Build history of the part. All positions in model axes, mm. Face numbers are marked on the shaded views. A direction names the side the tool comes from. Coordinates: 2 decimals unless noted, no trailing zeros. Order: outer loops, then holes, each group sorted by start corner. A loop starts at its lowest first (then second) coordinate and runs counter-clockwise, first axis right, second up. Notation, with made-up numbers: M 33.5,56 L 92.5,56 A20 cw 92.5,82 Z; hole C -32.5,73.5 d10. An arc over 180 degrees is marked long. Write item = value, one per line. Start each with the question number.
Q1. Pin check, flat tip, straight feed: P1, Ø5, axis at x = 4, z = 4, coming from the +Y side. Stop position of the tip, or through.
Q2. 3-axis set-ups, long thin cutter, end or side, ignore diameter. For the marked faces 1 and 2: which of +Z, -Z, +X, -X, +Y, -Y reach the whole face in a straight line?
Q3. Band-saw the part on D-D on x = 12.25. Write the cut outline in (y, z), plus the area to 3 significant figures.
Q4. Pull direction Z, two halves, no side cores. Call the marked faces 3, 4, 5 and 6: released by +Z, released by -Z, zero draft, split by the parting line, or undercut.
Q5. Band-saw the part on A-A on y = 9.25. Write the cut outline in (x, z), plus the area to 3 significant figures.
Q6. Band-saw the part on C-C on z = 4.25. Write the cut outline in (x, y), plus the area to 3 significant figures.
Q7. Drill centre lines: probe 1 along Z at (x, y) = (6.25, 6); probe 2 along Y at (x, z) = (6.35, 8); probe 3 along Y at (x, z) = (3, 1.25). Where is each one in solid material? Low to high.
Q8. Band-saw the part on B-B on x = 6.35. Write the cut outline in (y, z).
```python
from build123d import *

# Parameters (mm, degrees)
SKETCH1_R           = 0.5
BOSS_EXTRUDE1_DEPTH = 1
SKETCH2_W           = 12.7
SKETCH2_H           = 1
BOSS_EXTRUDE2_DEPTH = 6.35
SKETCH3_R           = 0.5
BOSS_EXTRUDE3_DEPTH = 1


with BuildPart() as part:
    # Sketch1 → Boss-Extrude1 (new body)
    with BuildSketch(Plane.XY):
        with BuildLine():
            Line((0, 0), (0, 19.05))
            ThreePointArc((0, 19.05), (6.35, 25.4), (12.7, 19.05))
            Line((12.7, 19.05), (12.7, 0))
            Line((12.7, 0), (0, 0))
        make_face()
        with Locations((6.35, 19.05)):
            Circle(SKETCH1_R, mode=Mode.SUBTRACT)
    extrude(amount=BOSS_EXTRUDE1_DEPTH)

    # Sketch2 → Boss-Extrude2 (add)
    with BuildSketch(Plane.XY.offset(1)):
        with Locations((6.35, 0.5)):
            Rectangle(SKETCH2_W, SKETCH2_H)
    extrude(amount=BOSS_EXTRUDE2_DEPTH)

    # Sketch3 → Boss-Extrude3 (add)
    with BuildSketch(Plane.XY.offset(7.35)):
        with BuildLine():
            Line((0, 0), (12.7, 0))
            Line((12.7, 0), (12.7, 19.05))
            ThreePointArc((12.7, 19.05), (6.35, 25.4), (0, 19.05))
            Line((0, 19.05), (0, 0))
        make_face()
        with Locations((6.35, 19.05)):
            Circle(SKETCH3_R, mode=Mode.SUBTRACT)
    extrude(amount=BOSS_EXTRUDE3_DEPTH)


solid = part.part
```
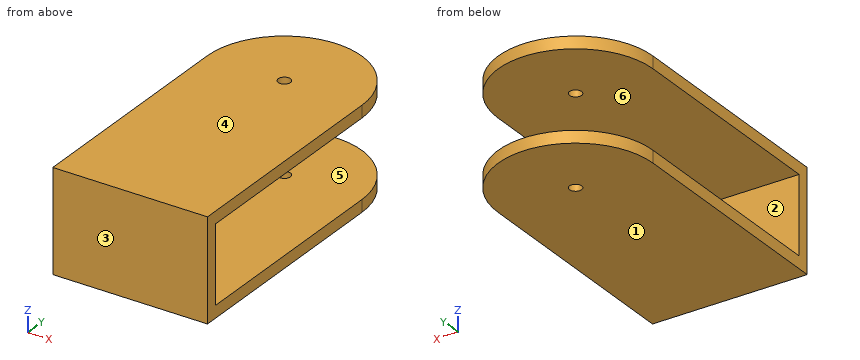
Recorded:
q1.P1 = 1
q2.face_1 = -Z, +X, -X, +Y, -Y
q2.face_2 = +X, -X, +Y
q3.outline = M 0,0 L 21.4,0 L 21.4,1 L 1,1 L 1,7.35 L 21.4,7.35 L 21.4,8.35 L 0,8.35 Z
q3.area = 49.1 mm2
q4.face_3 = zero draft
q4.face_4 = released by +Z
q4.face_5 = undercut
q4.face_6 = undercut
q5.outline = M 0,0 L 12.7,0 L 12.7,1 L 0,1 Z; M 0,7.35 L 12.7,7.35 L 12.7,8.35 L 0,8.35 Z
q5.area = 25.4 mm2
q6.outline = M 0,0 L 12.7,0 L 12.7,1 L 0,1 Z
q6.area = 12.7 mm2
q7.probe_1 = 0 to 1, 7.35 to 8.35
q7.probe_2 = 0 to 18.55, 19.55 to 25.4
q7.probe_3 = 0 to 1
q8.outline = M 0,0 L 18.55,0 L 18.55,1 L 1,1 L 1,7.35 L 18.55,7.35 L 18.55,8.35 L 0,8.35 Z; M 19.55,0 L 25.4,0 L 25.4,1 L 19.55,1 Z; M 19.55,7.35 L 25.4,7.35 L 25.4,8.35 L 19.55,8.35 Z
